The figure shows three views and two pictorial views of one solid part (mm, origin at its lowest corner). Answer the questions. Coordinates: 2 decimals unless noted, no trailing zeros. Order: outer loops, then holes, each group sorted by start corner. A loop starts at its lowest first (then second) coordinate and runs counter-clockwise, first axis right, second up. Notation, with made-up numbers: (1, 85) - (28, 85) arc R24 cw to (28, 103) - close; hole circle Ø1 at (8, -26). An arc over 180 degrees is marked (long way). Use one line per item in the form item = value.
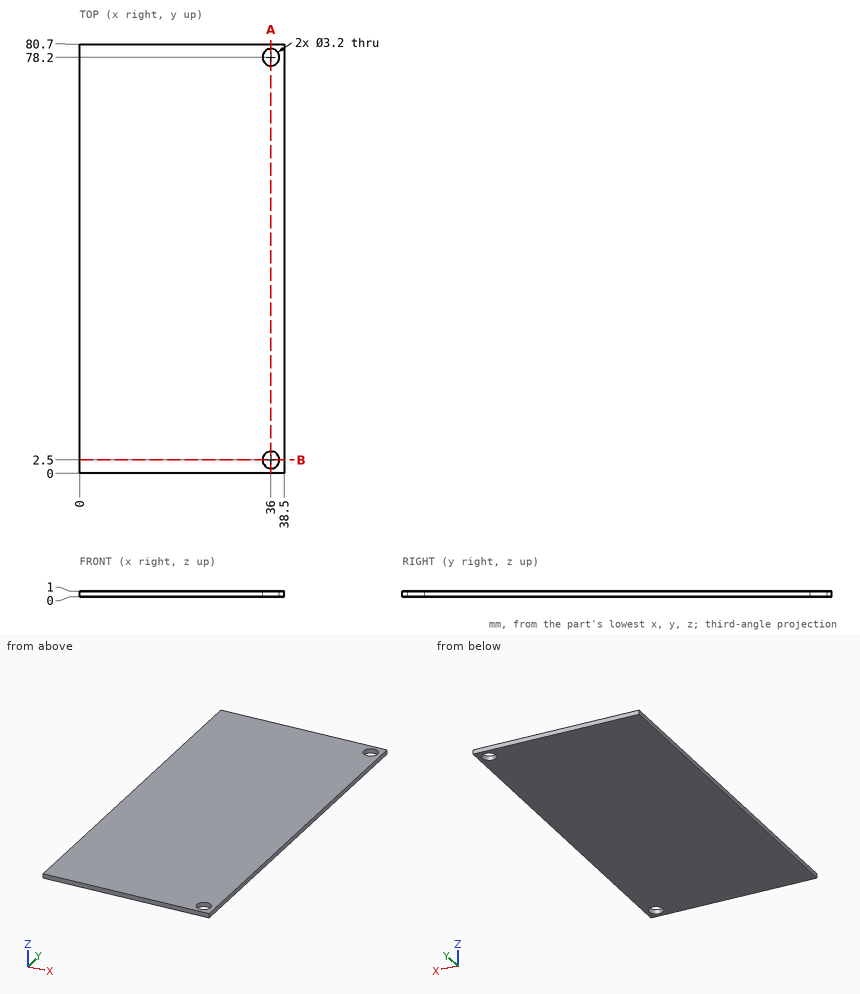
(1) Straight lines are drawn through the part: L1, parallel to Y at x = 36, z = 0.55; L2, parallel to X at y = 78.2, z = 0.25. For each, find the intervals that lie inside material, in ascending order.
Answer list:
L1 = 0 to 0.9, 4.1 to 76.6, 79.8 to 80.7
L2 = 0 to 34.4, 37.6 to 38.5
(2) Section A-A, the plane x = 36 is taken. Write down the section's boundary in (y, z), then the cut area to 3 significant figures.
Answer list:
outline = (0, 0) - (0.9, 0) - (0.9, 1) - (0, 1) - close; (4.1, 0) - (76.6, 0) - (76.6, 1) - (4.1, 1) - close; (79.8, 0) - (80.7, 0) - (80.7, 1) - (79.8, 1) - close
area = 74.3 mm2
(3) Section B-B, the plane y = 2.5 is taken. Write down the section's boundary in (x, z).
Answer list:
outline = (0, 0) - (34.4, 0) - (34.4, 1) - (0, 1) - close; (37.6, 0) - (38.5, 0) - (38.5, 1) - (37.6, 1) - close
